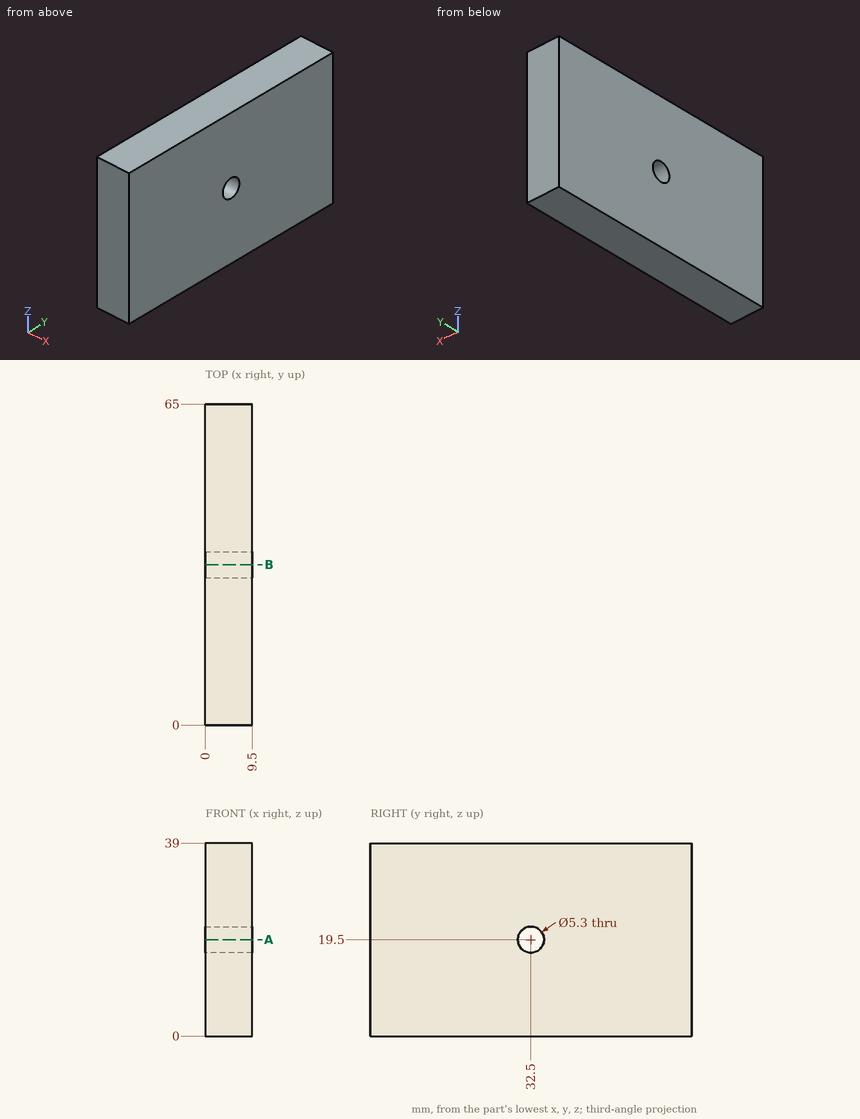
Here's the drawing with two shaded views (mm, measured from the low corner). I have some questions. Coordinates: 2 decimals unless noted, no trailing zeros. Write each loop counter-clockwise with the first axis right and the second up, starting at its lowest first coordinate (ties: lowest second). Pieces come first, ordered by that corner, then holes.
Item 1: I want a section at B-B on y = 32.5. Write out the boundary of the cut face in (x, z), and give its area (3 significant figures).
Item 2: If I drill on line 1 (Y direction, x = 3.75, z = 19.5); line 2 (Z direction, x = 4.5, y = 32.5); line 3 (Y direction, x = 6.75, z = 21.5), over which ranges is the centre line in solid material (lowest first)?
Item 3: I want a section at A-A on z = 19.5. Write out the boundary of the cut face in (x, y), and give its area (3 significant figures).
Item 4: Will this pin go through, and if not, where does the flat tip stop? pin 1 (6 mm diameter, centred on y = 43.5, z = 8, fed in from -X).
Findings below:
1. outline: (0, 0) - (9.5, 0) - (9.5, 16.85) - (0, 16.85) - close; (0, 22.15) - (9.5, 22.15) - (9.5, 39) - (0, 39) - close
1. area: 320 mm2
2. line 1: y = 0 to 29.85, 35.15 to 65
2. line 2: z = 0 to 16.85, 22.15 to 39
2. line 3: y = 0 to 30.76, 34.24 to 65
3. outline: (0, 0) - (9.5, 0) - (9.5, 29.85) - (0, 29.85) - close; (0, 35.15) - (9.5, 35.15) - (9.5, 65) - (0, 65) - close
3. area: 567 mm2
4. pin 1: stops at x = 0
